Geometry: final body of the model. Coordinates: model frame, mm. Face numbers are marked on the shaded views. A direction names the side the tool comes from. Coordinates: 2 decimals unless noted, no trailing zeros. Loops run counter-clockwise (first coordinate to the right, second up) from the corner with the lowest first, then second, coordinate; pieces in that order, holes last. Notation, with made-up numbers: (87, -15.75) - (111, -15.75) arc R7 ccw to (111, -6.75) - close; hole circle Ø6 at (48.25, -11.75). An arc over 180 degrees is marked (long way). Put each result on its own line as item: value. Start each with the question number.
1) Section A-A on x = 25. Output: boundary loops of the cut face in (y, z), and give its area (3 significant figures).
2) Section B-B on y = 61. Output: boundary loops of the cut face in (x, z) (3 decimals), and give its area (3 significant figures).
3) Material intervals for line 1 along X through (y, z) = (6.75, -11.5) (3 decimals); line 2 along X through (y, z) = (2, -11.5); line 3 along X through (y, z) = (69, -9.5) (3 decimals), sorted ascending. Write a range as from..to.
4) Contact query for flat-ended pins moving along their axis: pin 1 Ø2 at (y, z) = (107.5, -4) entering from -X; pin 2 Ø1 at (x, z) = (-14, -7.5) entering from +Y; pin 3 Ø1 at (x, y) = (-3.5, 50) entering from -Z; pin 4 Ø3.5 at (x, z) = (25, -11.5) entering from -Y. Output: stop coordinate, or through.
5) Reachability of the marked faces 1 and 2 from +Z, -Z, +X, -X, +Y, -Y: full face, straight path, thin tool, end or side. Return the list, or none.
6) Draft query along X for the marked faces 3, 4, 5 and 6. Return one class per face: +X half, -X half, draft (parallel to the pull), parting line (faces both ways), or undercut.
7) Section C-C on z = -11.5. Output: boundary loops of the cut face in (x, y) (3 decimals), and give its area (3 significant figures).
8) Section D-D on x = -11.5. Output: boundary loops of the cut face in (y, z), and give its area (3 significant figures).
```python
from build123d import *

# Parameters (mm, degrees)
SKETCH_1_W           = 70
SKETCH_1_H           = 43
EXTRUDE_1_DEPTH      = 10
SKETCH_21_R          = 3
CUT_EXTRUDE_12_DEPTH = 43.275879648
SKETCH_22_R          = 3
CUT_EXTRUDE_13_DEPTH = 43.275879648
SKETCH_46_W          = 15
SKETCH_46_H          = 12
EXTRUDE_4_DEPTH      = 200
SKETCH_76_W          = 7.65
SKETCH_76_H          = 200
CUT_EXTRUDE_37_DEPTH = 217.439367953
SKETCH_78_W          = 15
SKETCH_78_H          = 2
EXTRUDE_16_DEPTH     = 200
SKETCH_79_W          = 15
SKETCH_79_H          = 2
EXTRUDE_17_DEPTH     = 200
SKETCH_80_W          = 1.3
SKETCH_80_H          = 200
CUT_EXTRUDE_38_DEPTH = 215.359511102
SKETCH_83_W          = 7.65
SKETCH_83_H          = 12
CUT_EXTRUDE_39_DEPTH = 205.174557671
SKETCH_84_W          = 10
SKETCH_84_H          = 11
CUT_EXTRUDE_40_DEPTH = 218.195764231
SKETCH_82_W          = 15
SKETCH_82_H          = 16
EXTRUDE_19_DEPTH     = 10
SKETCH_85_W          = 70
SKETCH_85_H          = 15
CUT_EXTRUDE_41_DEPTH = 10
SKETCH_86_W          = 15
SKETCH_86_H          = 35
CUT_EXTRUDE_42_DEPTH = 25
SKETCH_87_W          = 15
SKETCH_87_H          = 16
EXTRUDE_20_DEPTH     = 5
SKETCH_88_W          = 15
SKETCH_88_H          = 28
CUT_EXTRUDE_43_DEPTH = 35
SKETCH_89_W          = 15
SKETCH_89_H          = 16
EXTRUDE_21_DEPTH     = 5
SKETCH_90_W          = 29.045295042
SKETCH_90_H          = 11
CUT_EXTRUDE_44_DEPTH = 20


with BuildPart() as part:
    # 草圖1 → 填料-伸長1 (new body)
    with BuildSketch(Plane(origin=(0, 0, 0), x_dir=(1, 0, 0), z_dir=(0, 1, 0))):
        Rectangle(SKETCH_1_W, SKETCH_1_H)
    extrude(amount=EXTRUDE_1_DEPTH)

    # 草圖21 → 除料-伸長12 (cut, through all)
    with BuildSketch(Plane(origin=(0, 10, 0), x_dir=(1, 0, 0), z_dir=(0, 1, 0))):
        with Locations(Location((-25, 11.5, 0), (0, 0, 270))):
            Circle(SKETCH_21_R)
    extrude(amount=-CUT_EXTRUDE_12_DEPTH, mode=Mode.SUBTRACT)

    # 草圖22 → 除料-伸長13 (cut, through all)
    with BuildSketch(Plane(origin=(0, 10, 0), x_dir=(1, 0, 0), z_dir=(0, 1, 0))):
        with Locations(Location((25, 11.5, 0), (0, 0, 270))):
            Circle(SKETCH_22_R)
    extrude(amount=-CUT_EXTRUDE_13_DEPTH, mode=Mode.SUBTRACT)

    # 草圖46 → 填料-伸長4 (add)
    with BuildSketch(Plane(origin=(0, 10, 0), x_dir=(1, 0, 0), z_dir=(0, 1, 0))):
        with Locations((0, 11.5)):
            Rectangle(SKETCH_46_W, SKETCH_46_H)
    extrude(amount=EXTRUDE_4_DEPTH)

    # 草圖76 → 除料-伸長37 (cut, through all)
    with BuildSketch(Plane(origin=(0, 0, -17.5), x_dir=(-1, 0, 0), z_dir=(0, 0, -1))):
        with Locations((0, 110)):
            Rectangle(SKETCH_76_W, SKETCH_76_H)
    extrude(amount=-CUT_EXTRUDE_37_DEPTH, mode=Mode.SUBTRACT)

    # 草圖78 → 填料-伸長16 (add)
    with BuildSketch(Plane(origin=(0, 10, 0), x_dir=(1, 0, 0), z_dir=(0, 1, 0))):
        with Locations((0, 4.5)):
            Rectangle(SKETCH_78_W, SKETCH_78_H)
    extrude(amount=EXTRUDE_16_DEPTH)

    # 草圖79 → 填料-伸長17 (add)
    with BuildSketch(Plane(origin=(0, 10, 0), x_dir=(1, 0, 0), z_dir=(0, 1, 0))):
        with Locations((0, 18.5)):
            Rectangle(SKETCH_79_W, SKETCH_79_H)
    extrude(amount=EXTRUDE_17_DEPTH)

    # 草圖80 → 除料-伸長38 (cut, through all)
    with BuildSketch(Plane.XY.offset(-3.5)):
        with Locations((0, 110)):
            Rectangle(SKETCH_80_W, SKETCH_80_H)
    extrude(amount=-CUT_EXTRUDE_38_DEPTH, mode=Mode.SUBTRACT)

    # 草圖83 → 除料-伸長39 (cut, through all)
    with BuildSketch(Plane(origin=(0, 10, 0), x_dir=(1, 0, 0), z_dir=(0, 1, 0))):
        with Locations((0, 11.5)):
            Rectangle(SKETCH_83_W, SKETCH_83_H)
    extrude(amount=-CUT_EXTRUDE_39_DEPTH, mode=Mode.SUBTRACT)

    # 草圖84 → 除料-伸長40 (cut, through all)
    with BuildSketch(Plane(origin=(0, 0, -21.5), x_dir=(-1, 0, 0), z_dir=(0, 0, -1))):
        Rectangle(SKETCH_84_W, SKETCH_84_H)
    extrude(amount=-CUT_EXTRUDE_40_DEPTH, mode=Mode.SUBTRACT)

    # 草圖82 → 填料-伸長19 (add)
    with BuildSketch(Plane(origin=(0, 210, 0), x_dir=(1, 0, 0), z_dir=(0, 1, 0))):
        with Locations((0, 11.5)):
            Rectangle(SKETCH_82_W, SKETCH_82_H)
    extrude(amount=EXTRUDE_19_DEPTH)

    # 草圖85 → 除料-伸長41 (cut)
    with BuildSketch(Plane(origin=(0, 10, 0), x_dir=(1, 0, 0), z_dir=(0, 1, 0))):
        with Locations((0, -14)):
            Rectangle(SKETCH_85_W, SKETCH_85_H)
    extrude(amount=-CUT_EXTRUDE_41_DEPTH, mode=Mode.SUBTRACT)

    # 草圖86 → 除料-伸長42 (cut)
    with BuildSketch(Plane.XY.offset(-3.5)):
        with Locations((0, 202.5)):
            Rectangle(SKETCH_86_W, SKETCH_86_H)
    extrude(amount=-CUT_EXTRUDE_42_DEPTH, mode=Mode.SUBTRACT)

    # 草圖87 → 填料-伸長20 (add)
    with BuildSketch(Plane(origin=(0, 185, 0), x_dir=(1, 0, 0), z_dir=(0, 1, 0))):
        with Locations((0, 11.5)):
            Rectangle(SKETCH_87_W, SKETCH_87_H)
    extrude(amount=EXTRUDE_20_DEPTH)

    # 草圖88 → 除料-伸長43 (cut)
    with BuildSketch(Plane(origin=(0, 0, -19.5), x_dir=(-1, 0, 0), z_dir=(0, 0, -1))):
        with Locations((0, 176)):
            Rectangle(SKETCH_88_W, SKETCH_88_H)
    extrude(amount=-CUT_EXTRUDE_43_DEPTH, mode=Mode.SUBTRACT)

    # 草圖89 → 填料-伸長21 (add)
    with BuildSketch(Plane(origin=(0, 162, 0), x_dir=(1, 0, 0), z_dir=(0, 1, 0))):
        with Locations((0, 11.5)):
            Rectangle(SKETCH_89_W, SKETCH_89_H)
    extrude(amount=EXTRUDE_21_DEPTH)

    # 草圖90 → 除料-伸長44 (cut)
    with BuildSketch(Plane.XY.offset(6.5)):
        Rectangle(SKETCH_90_W, SKETCH_90_H)
    extrude(amount=-CUT_EXTRUDE_44_DEPTH, mode=Mode.SUBTRACT)


solid = part.part
```
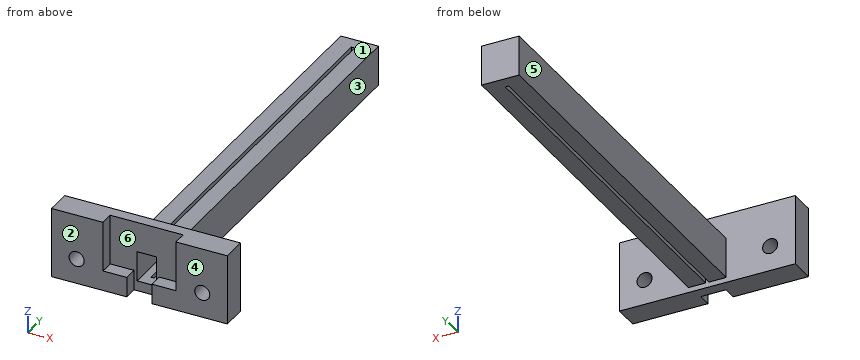
Answer block:
1. outline: (0, -21.5) - (10, -21.5) - (10, -14.5) - (0, -14.5) - close; (0, -8.5) - (10, -8.5) - (10, 6.5) - (0, 6.5) - close
1. area: 220 mm²
2. outline: (-7.5, -19.5) - (-0.65, -19.5) - (-0.65, -17.5) - (-3.825, -17.5) - (-3.825, -5.5) - (-0.65, -5.5) - (-0.65, -3.5) - (-7.5, -3.5) - close; (0.65, -19.5) - (7.5, -19.5) - (7.5, -3.5) - (0.65, -3.5) - (0.65, -5.5) - (3.825, -5.5) - (3.825, -17.5) - (0.65, -17.5) - close
2. area: 143 mm²
3. line 1: x = -35..-28, -22..-3.825, 3.825..22, 28..35
3. line 2: x = -35..-28, -22..-14.52, 14.52..22, 28..35
3. line 3: x = -7.5..-3.825, 3.825..7.5
4. pin 1: stops at x = -7.5
4. pin 2: stops at y = 10
4. pin 3: stops at z = -19.5
4. pin 4: passes through
5. face 1: +Z, +X, -X, +Y
5. face 2: +Z, -Z, +X, -X, -Y
6. face 3: +X half
6. face 4: draft
6. face 5: -X half
6. face 6: undercut
7. outline: (-35, 0) - (-28, 0) - (-28, 10) - (-35, 10) - close; (-22, 0) - (-14.523, 0) - (-14.523, 5.5) - (-3.825, 5.5) - (-3.825, 162) - (3.825, 162) - (3.825, 5.5) - (14.523, 5.5) - (14.523, 0) - (22, 0) - (22, 10) - (7.5, 10) - (7.5, 167) - (-7.5, 167) - (-7.5, 10) - (-22, 10) - close; (28, 0) - (35, 0) - (35, 10) - (28, 10) - close
7. area: 1,580 mm²
8. outline: (0, -21.5) - (10, -21.5) - (10, 6.5) - (5.5, 6.5) - (5.5, -13.5) - (0, -13.5) - close
8. area: 170 mm²
